Read the model definition and answer for the solid it produces. Units are mm, in the model's axes. Give positions to 0.01 mm unless a question says otherwise; leave off trailing zeros. Write each loop counter-clockwise with the first axis right and the second up, starting at its lowest first coordinate (ties: lowest second). Pieces come first, ordered by that corner, then holes. Notation, with made-up numbers: M 38.5,82 L 95.5,82 A23 cw 95.5,121 Z; hole C 60.5,68.25 d7. An arc over 180 degrees is marked long. Put each result on its own line as item: value.
Autodesk Inventor part; units mm, degrees
ref_plane "YZ Plane" through (0, 0, 0) normal (1, 0, 0) x (0, 1, 0)
ref_plane "XZ Plane" through (0, 0, 0) normal (0, 1, 0) x (-1, 0, 0)
ref_plane "XY Plane" through (0, 0, 0) normal (0, 0, 1) x (1, 0, 0)
sketch "Sketch1" plane through (0, 0, 0) normal (0, 1, 0) x (-1, 0, 0)
  circle A0 centre (0, 0) radius 1
  dimension "d0" = 2
extrude "Extrusion1" add sketch "Sketch1" along normal blind 6.2
fillet "Fillet1" radius 0.1 1 edges at (1, 6.2, 0)
sketch "Sketch2" plane through (0, 0, 0) normal (0, -1, 0) x (1, 0, 0)
  circle A0 centre (0, 0.7493) radius 0.1
  circle A1 centre (0, -0.7493) radius 0.1
  point P0 (0, 0)
  dimension "d4" = 0.2
  dimension "d5" = 0.2
  dimension "d6" = 0.7493
  dimension "d7" = 0.7493
extrude "Extrusion2" add sketch "Sketch2" along normal blind 3.2
properties part number "CFS-20632768EZBB_Watch_Crystal"
(1) Section B-B on z = 0 is taken. Determine the outline of the cut face in (x, y), and give its area (3 significant figures).
Result:
outline: M -1,0 L 1,0 L 1,6.1 A0.1 ccw 0.9,6.2 L -0.9,6.2 A0.1 ccw -1,6.1 Z
area: 12.4 mm²
(2) Section A-A on x = 0 is taken. Determine the outline of the cut face in (y, z), and give its area (3 significant figures).
Result:
outline: M -3.2,-0.85 L 0,-0.85 L 0,-1 L 6.1,-1 A0.1 ccw 6.2,-0.9 L 6.2,0.9 A0.1 ccw 6.1,1 L 0,1 L 0,0.85 L -3.2,0.85 L -3.2,0.65 L 0,0.65 L 0,-0.65 L -3.2,-0.65 Z
area: 13.7 mm²
(3) Straight lines are drawn through the part: line 1 along Z through (x, y) = (0.05, 0.75); line 2 along Y through (x, z) = (0.5, -0.7); line 3 along X through (y, z) = (-0.75, 0.75). For each, find the intervals that lie inside material, in ascending order. Write a range as from..to.
Result:
line 1: z = -1..1
line 2: y = 0..6.2
line 3: x = -0.1..0.1
(4) Section D-D on y = -1.75 is taken. Determine the outline of the cut face in (x, z).
Result:
outline: C 0,-0.75 d0.2; C 0,0.75 d0.2
(5) Section C-C on y = 2 is taken. Determine the outline of the cut face in (x, z).
Result:
outline: C 0,0 d2
